Part model, mm, in its own coordinate system. Give positions to 0.01 mm unless a question says otherwise; leave off trailing zeros. Order: outer loops, then holes, each group sorted by start corner. A loop starts at its lowest first (then second) coordinate and runs counter-clockwise, first axis right, second up.
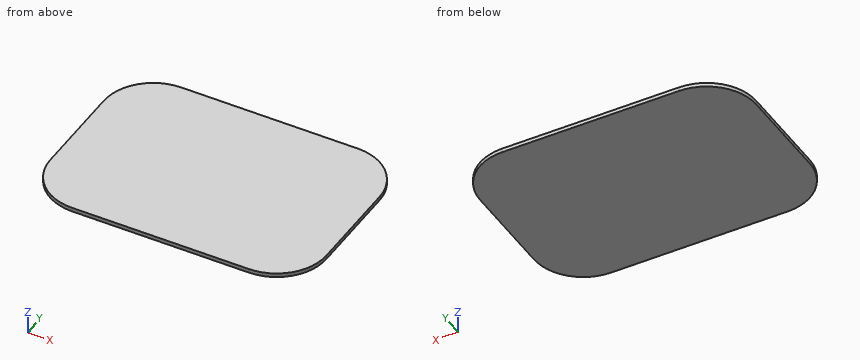
Autodesk Inventor part; units mm, degrees
ref_plane "YZ Plane" through (0, 0, 0) normal (1, 0, 0) x (0, 1, 0)
ref_plane "XZ Plane" through (0, 0, 0) normal (0, 1, 0) x (-1, 0, 0)
ref_plane "XY Plane" through (0, 0, 0) normal (0, 0, 1) x (1, 0, 0)
sketch "Sketch1" plane through (0, 0, 0) normal (0, 0, 1) x (1, 0, 0)
  line L0 (-44.5, -49) -> (44.5, -49)
  line L1 (69.5, -24) -> (69.5, 24)
  line L2 (44.5, 49) -> (-44.5, 49)
  line L3 (-69.5, 24) -> (-69.5, -24)
  line L4 (-69.5, -49) -> (69.5, 49) construction
  line L5 (69.5, -49) -> (-69.5, 49) construction
  arc A0 (69.5, 24) -> (44.5, 49) centre (44.5, 24) ccw
  arc A1 (44.5, -49) -> (69.5, -24) centre (44.5, -24) ccw
  arc A2 (-69.5, -24) -> (-44.5, -49) centre (-44.5, -24) ccw
  arc A3 (-44.5, 49) -> (-69.5, 24) centre (-44.5, 24) ccw
  point P0 (0, 0)
  dimension "d0" = 139
  dimension "d1" = 98
  dimension "d2" = 25
extrude "Extrusion1" add sketch "Sketch1" along normal mid plane 2
properties part number "Game_ColonyPort"
Item 1: Band-saw the part on A-A on z = 0.15. List the corners of the cut face in (x, y), plus the area to 3 significant figures.
Item 2: Band-saw the part on C-C on y = 40. List the corners of the cut face in (x, z).
Item 3: Band-saw the part on B-B on x = -58. List the corners of the cut face in (y, z).
Item 4: Drill centre lines: probe 1 along X at (y, z) = (44, -0.9); probe 2 along Y at (x, z) = (52, -0.25); probe 3 along X at (y, z) = (-25.5, 0.2). Where is each one in solid material? Low to high.
Item 5: Drop a flat-ended pin along its axis: P1, Ø1, axis at y = -30, z = -0.5, coming from the -X side. Give the stop position or say it passes through.
Working result:
1. outline: (-69.5, -24) arc R25 ccw to (-44.5, -49) - (44.5, -49) arc R25 ccw to (69.5, -24) - (69.5, 24) arc R25 ccw to (44.5, 49) - (-44.5, 49) arc R25 ccw to (-69.5, 24) - close
1. area: 13,100 mm2
2. outline: (-63.71, -1) - (63.71, -1) - (63.71, 1) - (-63.71, 1) - close
3. outline: (-45.04, -1) - (45.04, -1) - (45.04, 1) - (-45.04, 1) - close
4. probe 1: x = -59.5 to 59.5
4. probe 2: y = -47.85 to 47.85
4. probe 3: x = -69.45 to 69.45
5. P1: stops at x = -68.89
